```python
from build123d import *

# Parameters (mm, degrees)
F0_W     = 140
F0_H     = 124
F1_DEPTH = 5
F2_W     = 11
F2_H     = 124
F2_W_2   = 3
F3_DEPTH = 4
F4_R     = 60.5
F4_R_2   = 7.25
F4_R_3   = 1
F5_DEPTH = 2
F6_R     = 1
F7_DEPTH = 1
F8_R     = 1
F9_DEPTH = 1


with BuildPart() as f1:
    # F0 (on Top) → F1 (new body)
    with BuildSketch(Plane.XY):
        with Locations((2.145864, -1.898353)):
            Rectangle(F0_W, F0_H)
    extrude(amount=F1_DEPTH)

    # F2 (on face) → F3 (join)
    with BuildSketch(Plane.XY.offset(5)):
        with Locations((-62.354136, -1.898353)):
            Rectangle(F2_W, F2_H)
        with Locations((70.645864, -1.898353)):
            Rectangle(F2_W_2, F2_H)
    extrude(amount=F3_DEPTH)

    # F4 (on face) → F5 (cut)
    with BuildSketch(Plane.XY.offset(5)):
        with Locations((8.145864, -1.898353)):
            Circle(F4_R)
        with Locations((8.145864, -1.898353)):
            Circle(F4_R_2, mode=Mode.SUBTRACT)
        with Locations((8.145864, -1.898353)):
            Circle(F4_R_3)
    extrude(amount=-F5_DEPTH, mode=Mode.SUBTRACT)

    # F6 (on face) → F7 (cut)
    with BuildSketch(Plane.XZ.offset(63.898353)):
        with Locations((-62.854134, 4)):
            Circle(F6_R)
    extrude(amount=-F7_DEPTH, mode=Mode.SUBTRACT)

    # F8 (on face) → F9 (cut)
    with BuildSketch(Plane(origin=(0, 60.101647, 0), x_dir=(-1, 0, 0), z_dir=(0, 1, 0))):
        with Locations((62.854136, 4)):
            Circle(F8_R)
    extrude(amount=-F9_DEPTH, mode=Mode.SUBTRACT)


solid = f1.part
```
Geometry check sheet. Reference: the model listing, model coordinates, mm. A direction names the side the tool comes from. Give positions to 0.01 mm unless a question says otherwise; leave off trailing zeros. Order: outer loops, then holes, each group sorted by start corner. A loop starts at its lowest first (then second) coordinate and runs counter-clockwise, first axis right, second up.
1. Access from +Z, -Z, +X, -X, +Y, -Y to the whole of each face (thin tool, end or side, straight path). Record for faces 1 (the face through (-50, -20, 5)), 2 (the face through (1, -63.898, 2)), 3 (the face through (0.27, 58.087, 4.014)).
2. Section check C-C, the plane x = 57.5. Enter the section's corners in (y, z), and give its area (3 significant figures).
3. Section check D-D, the plane y = 13. Enter the section's corners in (x, z).
4. Section check A-A, the plane z = 6.5. Enter the section's corners in (x, y), and give its area (3 significant figures).
5. Release check for a two-part mould opening along X. For faces 4 (the face through (15.06, 0.28, 4.01)), 5 (the face through (1, 60.102, 2)), 6 (the face through (72.146, -3, 4)) record: pulls with the +X half, pulls with the -X half, needs draft (parallel to the pull), parting line crosses it, or undercut.
6. Thickness scan on L1, parallel to X at y = 52.5, z = 5.5; L2, parallel to Z at x = -17, y = -26; L3, parallel to Z at x = -42, y = 45. Record the ranges inside material, lowest first.
7. Gauge pin test, flat ends, axial feed: pin 1 Ø10 at (x, y) = (4, 24) entering from +Z; pin 2 Ø2.5 at (x, y) = (8.15, -1.9) entering from +Z; pin 3 Ø1.8 at (x, z) = (-62.85, 4) entering from +Y. Record the tip position at first contact, or that the pin passes through.
8. Section check B-B, the plane y = 34.5. Enter the section's corners in (x, z).
Values follow:
1. face 1: +Z, +Y, -Y
1. face 2: +Z, -Z, +X, -X, -Y
1. face 3: +Z
2. outline: (-63.9, 0) - (60.1, 0) - (60.1, 5) - (33.09, 5) - (33.09, 3) - (-36.89, 3) - (-36.89, 5) - (-63.9, 5) - close
2. area: 480 mm2
3. outline: (-67.85, 0) - (72.15, 0) - (72.15, 9) - (69.15, 9) - (69.15, 5) - (66.78, 5) - (66.78, 3) - (-50.49, 3) - (-50.49, 5) - (-56.85, 5) - (-56.85, 9) - (-67.85, 9) - close
4. outline: (-67.85, -63.9) - (-56.85, -63.9) - (-56.85, 60.1) - (-67.85, 60.1) - close; (69.15, -63.9) - (72.15, -63.9) - (72.15, 60.1) - (69.15, 60.1) - close
4. area: 1,740 mm2
5. face 4: undercut
5. face 5: needs draft
5. face 6: pulls with the +X half
6. L1: x = -67.85 to -56.85, 69.15 to 72.15
6. L2: z = 0 to 3
6. L3: z = 0 to 5
7. pin 1: stops at z = 3
7. pin 2: stops at z = 5
7. pin 3: stops at y = 59.1
8. outline: (-67.85, 0) - (72.15, 0) - (72.15, 9) - (69.15, 9) - (69.15, 5) - (56.47, 5) - (56.47, 3) - (-40.18, 3) - (-40.18, 5) - (-56.85, 5) - (-56.85, 9) - (-67.85, 9) - close
